```python
from build123d import *

# Parameters (mm, degrees)
BOSS_EXTRUDE3_DEPTH = 5
CHAMFER3_SIZE       = 3


with BuildPart() as part:
    # Sketch7 → Boss-Extrude3 (new body)
    with BuildSketch(Plane.XY):
        Polygon((-298.426339507, 70), (-284.496051046, 108), (-293.092548077, 108), (-293.092548077, 104.25), (-288.000901442, 104.25), (-299.181790865, 73.75), (-329.592548077, 73.75), (-329.592548077, 104.25), (-324.092548077, 104.25), (-324.092548077, 108), (-333.092548077, 108), (-333.092548077, 70), align=None)
    extrude(amount=BOSS_EXTRUDE3_DEPTH)

    # Chamfer3
    chamfer3_edges = [part.edges().sort_by_distance(p)[0] for p in [
        (-293.092548077, 108, 2.5),
        (-324.092548077, 108, 2.5),
    ]]
    chamfer(chamfer3_edges, length=CHAMFER3_SIZE)


solid = part.part
```
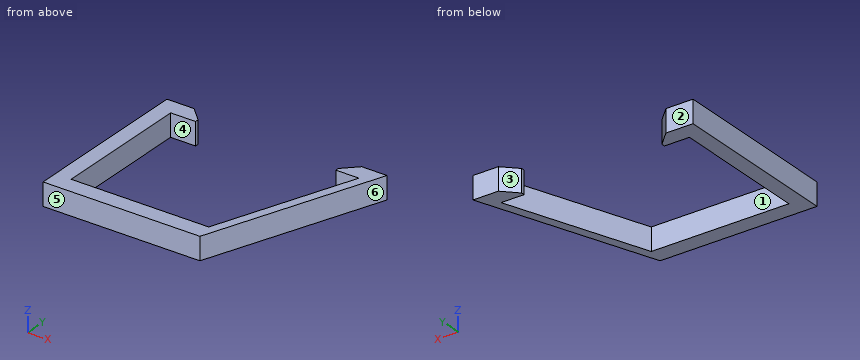
CAD build for the part. Positions are in the model's coordinates, mm. Face numbers are marked on the shaded views. A direction names the side the tool comes from. Give positions to 0.01 mm unless a question says otherwise; leave off trailing zeros. Loops run counter-clockwise (first coordinate to the right, second up) from the corner with the lowest first, then second, coordinate; pieces in that order, holes last. Notation, with made-up numbers: (74, 68) -> (103, 68) arc R11 cw to (103, 78) -> close; hole circle Ø1 at (-30, 4.25). An arc over 180 degrees is marked (long way). Use a Markdown table: item, result.
1. Slice it at A-A (y = 81). List the corners of the cut face in (x, z).
Check result:
| item | result |
|---|---|
| outline | (-333.09, 0) -> (-329.59, 0) -> (-329.59, 5) -> (-333.09, 5) -> close; (-296.52, 0) -> (-294.39, 0) -> (-294.39, 5) -> (-296.52, 5) -> close |
2. Which spindle directions (+Z, -Z, +X, -X, +Y, -Y) get a long thin tool onto all of the face, cutting with end or side? Do the marked faces 1, 2 and 3. Say none if no direction does.
Check result:
| item | result |
|---|---|
| face 1 | +Z, -Z |
| face 2 | +Z, -Z, +X, -X, +Y |
| face 3 | +Z, -Z, +Y |
3. Slice it at C-C (z = 1.1). List the corners of the cut face in (x, y), plus the area to 3 significant figures.
Check result:
| item | result |
|---|---|
| outline | (-333.09, 70) -> (-298.43, 70) -> (-284.5, 108) -> (-290.09, 108) -> (-293.09, 105) -> (-293.09, 104.25) -> (-288, 104.25) -> (-299.18, 73.75) -> (-329.59, 73.75) -> (-329.59, 104.25) -> (-324.09, 104.25) -> (-324.09, 105) -> (-327.09, 108) -> (-333.09, 108) -> close |
| area | 359 mm^2 |
4. Slice it at D-D (x = -294). List the corners of the cut face in (y, z), plus the area to 3 significant figures.
Check result:
| item | result |
|---|---|
| outline | (82.07, 0) -> (87.89, 0) -> (87.89, 5) -> (82.07, 5) -> close |
| area | 29.1 mm^2 |
5. Slice it at B-B (x = -325.5). List the corners of the cut face in (y, z).
Check result:
| item | result |
|---|---|
| outline | (70, 0) -> (73.75, 0) -> (73.75, 5) -> (70, 5) -> close; (104.25, 0) -> (106.41, 0) -> (106.41, 5) -> (104.25, 5) -> close |
6. Mould opens along X. For the marked faces 4, 5 and 6 say: pulls with the +X half, pulls with the -X half, needs draft (parallel to the pull), parting line crosses it, or undercut.
Check result:
| item | result |
|---|---|
| face 4 | undercut |
| face 5 | needs draft |
| face 6 | pulls with the +X half |
7. Flat gauge pins, fed straight in: pin 1 (1 mm diameter, centred on x = -303.5, z = 0.5, fed in from +Y); pin 2 (1.5 mm diameter, centred on y = 84, z = 2.5, fed in from +X). Where does each tip first touch, or does it go through?
Check result:
| item | result |
|---|---|
| pin 1 | stops at y = 73.75 |
| pin 2 | stops at x = -293.02 |
8. Wall check: L1, parallel to X at y = 98.5, z = 4.2; L2, parallel to X at y = 106.5, z = 2.9; L3, parallel to Y at x = -302.5, z = 4.65. Give the ranges that are in metal, low to high. Write a range as [from, to].
Check result:
| item | result |
|---|---|
| L1 | x = [-333.09, -329.59], [-290.11, -287.98] |
| L2 | x = [-333.09, -325.59], [-291.59, -285.05] |
| L3 | y = [70, 73.75] |
